```python
from build123d import *

# Parameters (mm, degrees)
CROQUIS1_R              = 5
SALIENTE_EXTRUIR1_DEPTH = 50
CHAFL_N1_SIZE           = 1
CROQUIS4_W              = 1.5
CROQUIS4_H              = 1.5
CROQUIS5_OUTSIDE_W      = 32.2
CROQUIS5_OUTSIDE_H      = 32.2
CROQUIS5_OUTSIDE_R      = 4
CORTAR_EXTRUIR2_DEPTH   = 28
CHAFL_N3_SIZE           = 1


with BuildPart() as part:
    # Croquis1 → Saliente-Extruir1 (new, symmetric)
    with BuildSketch(Plane.XY):
        Circle(CROQUIS1_R)
    extrude(amount=SALIENTE_EXTRUIR1_DEPTH, both=True)

    # Chaflán1
    chafl_n1_edges = [part.edges().sort_by_distance(p)[0] for p in [
        (-5, 0, -50),
    ]]
    chamfer(chafl_n1_edges, length=CHAFL_N1_SIZE)

    # Croquis4 → Cortar-Revolución2 (revolve, cut)
    with BuildSketch(Plane(origin=(0, 0, 0), x_dir=(1, 0, 0), z_dir=(0, 1, 0))):
        with Locations((5, 18.25)):
            Rectangle(CROQUIS4_W, CROQUIS4_H)
        with Locations((5, -19.25)):
            Rectangle(CROQUIS4_W, CROQUIS4_H)
    revolve(axis=Axis((0, 0, 0), (0, 0, -1)), mode=Mode.SUBTRACT)

    # Croquis5 outside → Cortar-Extruir2 (cut)
    with BuildSketch(Plane.XY.offset(50)):
        Rectangle(CROQUIS5_OUTSIDE_W, CROQUIS5_OUTSIDE_H)
        Circle(CROQUIS5_OUTSIDE_R, mode=Mode.SUBTRACT)
    extrude(amount=-CORTAR_EXTRUIR2_DEPTH, mode=Mode.SUBTRACT)

    # Chaflán3
    chafl_n3_edges = [part.edges().sort_by_distance(p)[0] for p in [
        (-4, 0, 50),
    ]]
    chamfer(chafl_n3_edges, length=CHAFL_N3_SIZE)


solid = part.part
```
Verification items for the finished model (mm, model axes). A direction names the side the tool comes from. Coordinates: 2 decimals unless noted, no trailing zeros. Loops run counter-clockwise (first coordinate to the right, second up) from the corner with the lowest first, then second, coordinate; pieces in that order, holes last. Notation, with made-up numbers: (16, 32) - (68, 32) arc R20 cw to (68, 71) - close; hole circle Ø5 at (55, 58.5). An arc over 180 degrees is marked (long way). Return JSON: item names as keys, results as strings.
1. Thickness scan on L1, parallel to Z at x = -3.75, y = -3; L2, parallel to Y at x = 0.25, z = 34.5; L3, parallel to Y at x = -0.25, z = -15. Record the ranges inside material, lowest first.
Established:
{"L1": "z = -49.2 to -19, -17.5 to 18.5, 20 to 22", "L2": "y = -3.99 to 3.99", "L3": "y = -4.99 to 4.99"}
2. Section check C-C, the plane z = -13.5. Record the boundary of the cut face in (x, y).
Established:
{"outline": "circle Ø10 at (0, 0)"}
3. Section check A-A, the plane y = 0. Record the boundary of the cut face in (x, z), then the cut area to 4 significant figures.
Established:
{"outline": "(-5, -49) - (-4, -50) - (4, -50) - (5, -49) - (5, -19) - (4.25, -19) - (4.25, -17.5) - (5, -17.5) - (5, 18.5) - (4.25, 18.5) - (4.25, 20) - (5, 20) - (5, 22) - (4, 22) - (4, 49) - (3, 50) - (-3, 50) - (-4, 49) - (-4, 22) - (-5, 22) - (-5, 20) - (-4.25, 20) - (-4.25, 18.5) - (-5, 18.5) - (-5, -17.5) - (-4.25, -17.5) - (-4.25, -19) - (-5, -19) - close", "area": "937.5 mm2"}
4. Tool access check on faces 1 (the flat face through (2, 4, -19)), 2 (the cylindrical face through (-1.08, -4.88, -33.79)), 3 (the cylindrical face through (-0.867, -3.905, 35.689)). Record the directions out of +Z, -Z, +X, -X, +Y, -Y that give a thin tool (end or side, any length) a straight path to the whole face; none if there is none.
Established:
{"face 1": "none", "face 2": "+Z, -Z", "face 3": "+Z"}
5. Go/stop test with flat-tipped pins: pin 1 (3 mm diameter, centred on x = -0.5, z = 8.5, fed in from +Y); pin 2 (3 mm diameter, centred on x = 3.5, z = 8, fed in from -Y); pin 3 (1.5 mm diameter, centred on y = -1, z = 4, fed in from -X); pin 4 (1.5 mm diameter, centred on x = -2, z = -29, fed in from +Y). Record where each tip stops, or that it passes through.
Established:
{"pin 1": "stops at y = 5", "pin 2": "stops at y = -4.58", "pin 3": "stops at x = -4.99", "pin 4": "stops at y = 4.84"}
6. Section check D-D, the plane z = 42. Record the boundary of the cut face in (x, y).
Established:
{"outline": "circle Ø8 at (0, 0)"}
